```python
from build123d import *

# Parameters (mm, degrees)
PAD_DEPTH       = 120
SKETCH001_W     = 10
SKETCH001_H     = 60
PAD001_DEPTH    = 50
POCKET_DEPTH    = 10
POCKET001_DEPTH = 5
POCKET002_DEPTH = 5


with BuildPart() as part:
    # Sketch → Pad (new body)
    with BuildSketch(Plane.XZ):
        with BuildLine():
            Line((-40, 0), (40, 0))
            Line((40, 0), (40, 36))
            Line((40, 36), (30, 36))
            ThreePointArc((-30, 36), (0, 6), (30, 36))
            Line((-40, 36), (-30, 36))
            Line((-40, 0), (-40, 36))
        make_face()
    extrude(amount=PAD_DEPTH)

    # Sketch001 (on Face5 of Pad) → Pad001 (join)
    with BuildSketch(Plane(origin=(0, 0, 36), x_dir=(-1, 0, 0), z_dir=(0, 0, 1))):
        with Locations((-35, 90)):
            Rectangle(SKETCH001_W, SKETCH001_H)
        with Locations((35, 90)):
            Rectangle(SKETCH001_W, SKETCH001_H)
    extrude(amount=PAD001_DEPTH)

    # Sketch002 (on Face14 of Pad001) → Pocket (cut)
    with BuildSketch(Plane(origin=(0, 0, 86), x_dir=(-1, 0, 0), z_dir=(0, 0, 1))):
        with BuildLine():
            ThreePointArc((33, 86), (35, 84), (37, 86))
            Line((37, 86), (37, 94))
            ThreePointArc((37, 94), (35, 96), (33, 94))
            Line((33, 86), (33, 94))
        make_face()
        with BuildLine():
            ThreePointArc((-37, 86), (-35, 84), (-33, 86))
            Line((-33, 86), (-33, 94))
            ThreePointArc((-33, 94), (-35, 96), (-37, 94))
            Line((-37, 86), (-37, 94))
        make_face()
    extrude(amount=-POCKET_DEPTH, mode=Mode.SUBTRACT)

    # Sketch003 (on Face7 of Pocket) → Pocket001 (cut)
    with BuildSketch(Plane(origin=(-40, 0, 0), x_dir=(0, 0, -1), z_dir=(-1, 0, 0))):
        with BuildLine():
            ThreePointArc((-80, 86), (-78, 84), (-76, 86))
            Line((-76, 86), (-76, 94))
            ThreePointArc((-76, 94), (-78, 96), (-80, 94))
            Line((-80, 86), (-80, 94))
        make_face()
    extrude(amount=-POCKET001_DEPTH, mode=Mode.SUBTRACT)

    # Sketch004 (on Face9 of Pocket001) → Pocket002 (cut)
    with BuildSketch(Plane(origin=(40, 0, 0), x_dir=(0, 0, 1), z_dir=(1, 0, 0))):
        with BuildLine():
            ThreePointArc((80, 94), (78, 96), (76, 94))
            Line((76, 94), (76, 86))
            ThreePointArc((76, 86), (78, 84), (80, 86))
            Line((80, 94), (80, 86))
        make_face()
    extrude(amount=-POCKET002_DEPTH, mode=Mode.SUBTRACT)


solid = part.part
```
Read the model definition and answer for the solid it produces. Units are mm, in the model's axes. A direction names the side the tool comes from. Give positions to 0.01 mm unless a question says otherwise; leave off trailing zeros. Loops run counter-clockwise (first coordinate to the right, second up) from the corner with the lowest first, then second, coordinate; pieces in that order, holes last.
Item 1: For faces 3 (the flat face through (-39, -90, 80)), 4 (the cylindrical face through (-35, -96, 81)), 5 (the flat face through (-35, -30, 36)), determine the directions among +Z, -Z, +X, -X, +Y, -Y from which every point of the face is accessible in a straight line to the end or side of a thin tool.
Item 2: The mould has two halves that part along X. Classify faces 1 (the flat face through (-30, -90, 61)), 2 (the flat face through (35, -60, 61)): released by +X, released by -X, zero draft, split by the parting line, or undercut.
Item 3: Each of these flat-tipped pins is pushed along its axis until it touches: pin 1 Ø11 at (x, y) = (-35.5, -25) entering from +Z; pin 2 Ø1 at (x, z) = (31, 35) entering from +Y; pin 3 Ø11 at (x, z) = (34.5, 69.5) entering from +Y; pin 4 Ø1 at (x, y) = (18, -35) entering from +Z. Where does it stop, or does it pass through?
Item 4: Find the intervals of material crossed by line 1 along X through (y, z) = (-107.5, 79.5); line 2 along Y through (x, z) = (-36, 79); line 3 along X through (y, z) = (-52.5, 17), in increasing order.
Item 5: The part is cut by section A-A (y = -90.5). Write down the section's boundary in (x, z).
Item 6: The part is cut by section B-B (z = 78). Write down the section's boundary in (x, y).
Item 7: The part is cut by section C-C (y = -75). Write down the section's boundary in (x, z).
Item 8: The part is cut by section D-D (x = 0). Write down the section's boundary in (y, z).
Taken from the geometry:
1. face 3: -X
1. face 4: +Z
1. face 5: +Z, +X, -X, +Y
2. face 1: undercut
2. face 2: zero draft
3. pin 1: stops at z = 36
3. pin 2: stops at y = 0
3. pin 3: stops at y = -60
3. pin 4: stops at z = 12.38
4. line 1: x = -40 to -30, 30 to 40
4. line 2: y = -120 to -95.73, -84.27 to -60
4. line 3: x = -40 to -23.22, 23.22 to 40
5. outline: (-40, 0) - (40, 0) - (40, 76) - (33, 76) - (33, 86) - (30, 86) - (30, 36) arc R30 cw to (-30, 36) - (-30, 86) - (-33, 86) - (-33, 76) - (-40, 76) - close; (-40, 80) - (-37, 80) - (-37, 86) - (-40, 86) - close; (37, 80) - (40, 80) - (40, 86) - (37, 86) - close
6. outline: (-40, -120) - (-30, -120) - (-30, -60) - (-40, -60) - (-40, -84) - (-35, -84) arc R2 cw to (-33, -86) - (-33, -94) arc R2 cw to (-35, -96) - (-40, -96) - close; (30, -120) - (40, -120) - (40, -96) - (35, -96) arc R2 cw to (33, -94) - (33, -86) arc R2 cw to (35, -84) - (40, -84) - (40, -60) - (30, -60) - close
7. outline: (-40, 0) - (40, 0) - (40, 86) - (30, 86) - (30, 36) arc R30 cw to (-30, 36) - (-30, 86) - (-40, 86) - close
8. outline: (-120, 0) - (0, 0) - (0, 6) - (-120, 6) - close
